Could you check a few things on this model? Use its own coordinates, in mm. Face numbers are marked on the shaded views. Round coordinates to 2 decimals unless told otherwise and drop trailing zeros. Loops run counter-clockwise (first coordinate to the right, second up) from the corner with the lowest first, then second, coordinate; pieces in that order, holes last. Notation, with made-up numbers: M 38.5,21 L 52.5,21 A16 cw 52.5,26 Z; hole C 49.25,7 d8. An arc over 180 degrees is marked long. Return JSON: item names as keys, results as strings. Group by question number.
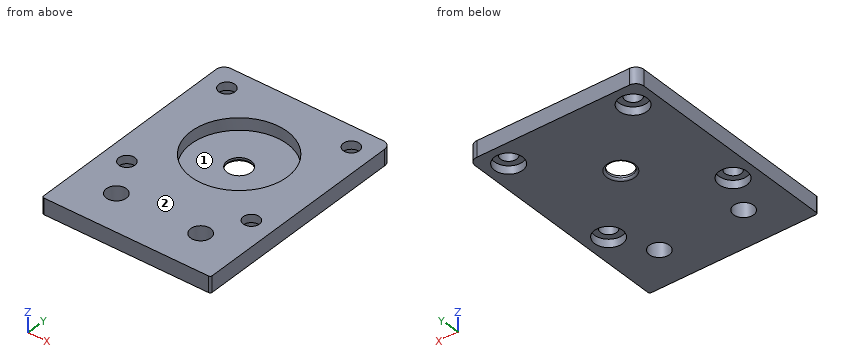
```python
from build123d import *

# Parameters (mm, degrees)
SKETCH1_R           = 2.999999999
BOSS_EXTRUDE1_DEPTH = 4
SKETCH5_R           = 12
CUT_EXTRUDE1_DEPTH  = 3
FILLET1_R           = 2
FILLET2_R           = 0.5
FILLET3_R           = 0.5
SKETCH6_R           = 2.5
CUT_EXTRUDE2_DEPTH  = 10
SKETCH7_R           = 2
CUT_EXTRUDE3_DEPTH  = 10
SKETCH8_R           = 3.5
CUT_EXTRUDE4_DEPTH  = 2


with BuildPart() as part:
    # Sketch1 → Boss-Extrude1 (new body)
    with BuildSketch(Plane.XY):
        Polygon((0, 0), (42, 0), (42, 51.371572875), (42, 56), (37.371572875, 56), (4.628427125, 56), (0, 56), align=None)
        with Locations((21, 35)):
            Circle(SKETCH1_R, mode=Mode.SUBTRACT)
    extrude(amount=BOSS_EXTRUDE1_DEPTH)

    # Sketch5 → Cut-Extrude1 (cut)
    with BuildSketch(Plane.XY.offset(4)):
        with Locations((21, 35)):
            Circle(SKETCH5_R)
    extrude(amount=-CUT_EXTRUDE1_DEPTH, mode=Mode.SUBTRACT)

    # Fillet1
    fillet1_edges = [part.edges().sort_by_distance(p)[0] for p in [
        (0, 56, 2),
        (42, 56, 2),
    ]]
    fillet(fillet1_edges, radius=FILLET1_R)

    # Fillet2
    fillet2_edges = [part.edges().sort_by_distance(p)[0] for p in [
        (42, 0, 2),
        (0, 0, 2),
    ]]
    fillet(fillet2_edges, radius=FILLET2_R)

    # Fillet3
    fillet3_edges = [part.edges().sort_by_distance(p)[0] for p in [
        (18.000000001, 35, 0),
    ]]
    fillet(fillet3_edges, radius=FILLET3_R)

    # Sketch6 → Cut-Extrude2 (cut)
    with BuildSketch(Plane.XY.offset(4)):
        with Locations((10.5, 10)):
            Circle(SKETCH6_R)
        with Locations((31.5, 10)):
            Circle(SKETCH6_R)
    extrude(amount=-CUT_EXTRUDE2_DEPTH, mode=Mode.SUBTRACT)

    # Sketch7 → Cut-Extrude3 (cut)
    with BuildSketch(Plane.XY.offset(4)):
        with Locations((5.5, 50.5)):
            Circle(SKETCH7_R)
        with Locations((5.5, 19.5)):
            Circle(SKETCH7_R)
        with Locations((36.5, 19.5)):
            Circle(SKETCH7_R)
        with Locations((36.5, 50.5)):
            Circle(SKETCH7_R)
    extrude(amount=-CUT_EXTRUDE3_DEPTH, mode=Mode.SUBTRACT)

    # Sketch8 → Cut-Extrude4 (cut)
    with BuildSketch(Plane(origin=(0, 0, 0), x_dir=(-1, 0, 0), z_dir=(0, 0, -1))):
        with Locations((-36.5, 50.5)):
            Circle(SKETCH8_R)
        with Locations((-36.5, 19.5)):
            Circle(SKETCH8_R)
        with Locations((-5.5, 19.5)):
            Circle(SKETCH8_R)
        with Locations((-5.5, 50.5)):
            Circle(SKETCH8_R)
    extrude(amount=-CUT_EXTRUDE4_DEPTH, mode=Mode.SUBTRACT)


solid = part.part
```
1. I need wall thicknesses on probe 1 along Y at (x, z) = (36.5, 3); probe 2 along Y at (x, z) = (10, 3.2); probe 3 along X at (y, z) = (17, 0.3). Which ranges of each line are inside material? Lowest first, please.
2. We'd pull the mould along Y, two halves only. Please class the marked faces 1 and 2: +Y half, -Y half, draft (parallel to the pull), parting line (faces both ways), or undercut.
3. If we section it at A-A, the plane y = 50.5: Please give me the cut outline in (x, z), then the cut area to 3 significant figures.
4. I'm going to push flat-ended pins straight in: pin 1 Ø2 at (x, y) = (7, 51) entering from -Z; pin 2 Ø3 at (x, y) = (28.5, 33.5) entering from +Z. Where does each tip first touch, or does it pass through?
5. If we section it at D-D, the plane y = 35: Please give me the cut outline in (x, z).
6. If we section it at B-B, the plane x = 21: Please give me the cut outline in (y, z).
7. If we section it at C-C, the plane z = 3.4: Please give me the cut outline in (x, y), then the cut area to 3 significant figures.
Geometry results:
{
 "1": {"probe 1": "0 to 17.5, 21.5 to 48.5, 52.5 to 56", "probe 2": "0 to 7.55, 12.45 to 30.2, 39.8 to 56", "probe 3": "0 to 3.05, 7.95 to 34.05, 38.95 to 42"},
 "2": {"face 1": "undercut", "face 2": "draft"},
 "3": {"outline": "M 0,0 L 2,0 L 2,2 L 3.5,2 L 3.5,4 L 0,4 Z; M 7.5,2 L 9,2 L 9,0 L 33,0 L 33,2 L 34.5,2 L 34.5,4 L 7.5,4 Z; M 38.5,2 L 40,2 L 40,0 L 42,0 L 42,4 L 38.5,4 Z", "area": "124 mm^2"},
 "4": {"pin 1": "z = 2", "pin 2": "z = 1"},
 "5": {"outline": "M 0,0 L 17.5,0 A0.5 ccw 18,0.5 L 18,1 L 9,1 L 9,4 L 0,4 Z; M 24,0.5 A0.5 ccw 24.5,0 L 42,0 L 42,4 L 33,4 L 33,1 L 24,1 Z"},
 "6": {"outline": "M 0,0 L 31.5,0 A0.5 ccw 32,0.5 L 32,1 L 23,1 L 23,4 L 0,4 Z; M 38,0.5 A0.5 ccw 38.5,0 L 56,0 L 56,4 L 47,4 L 47,1 L 38,1 Z"},
 "7": {"outline": "M 0,0.5 A0.5 ccw 0.5,0 L 41.5,0 A0.5 ccw 42,0.5 L 42,54 A2 ccw 40,56 L 2,56 A2 ccw 0,54 Z; hole C 5.5,19.5 d4; hole C 5.5,50.5 d4; hole C 10.5,10 d5; hole C 21,35 d24; hole C 31.5,10 d5; hole C 36.5,19.5 d4; hole C 36.5,50.5 d4", "area": "1,810 mm^2"}
}
